The listing builds one solid part. Answer for the finished solid, in the listing's coordinates (mm). A direction names the side the tool comes from. Coordinates: 2 decimals unless noted, no trailing zeros. Order: outer loops, then holes, each group sorted by start corner. A loop starts at its lowest first (then second) coordinate and runs counter-clockwise, first axis right, second up.
```python
from build123d import *

# Parameters (mm, degrees)
SKETCH1_W           = 112.5
SKETCH1_H           = 21.6
SKETCH1_R           = 2
BOSS_EXTRUDE1_DEPTH = 13
SKETCH2_W           = 8
SKETCH2_H           = 21.6
CUT_EXTRUDE1_DEPTH  = 5.8
FILLET1_R           = 1


with BuildPart() as part:
    # Sketch1 → Boss-Extrude1 (new body)
    with BuildSketch(Plane.XY):
        Rectangle(SKETCH1_W, SKETCH1_H)
        with Locations(Location((-52.5, 4, 0), (0, 0, 180))):
            Circle(SKETCH1_R, mode=Mode.SUBTRACT)
        with Locations(Location((52.5, 4, 0), (0, 0, 180))):
            Circle(SKETCH1_R, mode=Mode.SUBTRACT)
        with Locations(Location((52.5, -4, 0), (0, 0, 180))):
            Circle(SKETCH1_R, mode=Mode.SUBTRACT)
        with Locations(Location((-52.5, -4, 0), (0, 0, 180))):
            Circle(SKETCH1_R, mode=Mode.SUBTRACT)
    extrude(amount=BOSS_EXTRUDE1_DEPTH)

    # Sketch2 → Cut-Extrude1 (cut)
    with BuildSketch(Plane.XY.offset(13)):
        with Locations((-42.75, 0)):
            Rectangle(SKETCH2_W, SKETCH2_H)
        with Locations((-52.25, 0)):
            Rectangle(SKETCH2_W, SKETCH2_H)
        with Locations((-33.25, 0)):
            Rectangle(SKETCH2_W, SKETCH2_H)
        with Locations((-23.75, 0)):
            Rectangle(SKETCH2_W, SKETCH2_H)
        with Locations((-14.25, 0)):
            Rectangle(SKETCH2_W, SKETCH2_H)
        with Locations((-4.75, 0)):
            Rectangle(SKETCH2_W, SKETCH2_H)
        with Locations((4.75, 0)):
            Rectangle(SKETCH2_W, SKETCH2_H)
        with Locations((14.25, 0)):
            Rectangle(SKETCH2_W, SKETCH2_H)
        with Locations((23.75, 0)):
            Rectangle(SKETCH2_W, SKETCH2_H)
        with Locations((33.25, 0)):
            Rectangle(SKETCH2_W, SKETCH2_H)
        with Locations((42.75, 0)):
            Rectangle(SKETCH2_W, SKETCH2_H)
        with Locations((52.25, 0)):
            Rectangle(SKETCH2_W, SKETCH2_H)
    extrude(amount=-CUT_EXTRUDE1_DEPTH, mode=Mode.SUBTRACT)

    # Fillet1
    fillet1_edges = [part.edges().sort_by_distance(p)[0] for p in [
        (47.5, 10.8, 13),
        (38, 10.8, 13),
        (28.5, 10.8, 13),
        (19, 10.8, 13),
        (9.5, 10.8, 13),
        (0, 10.8, 13),
        (-9.5, 10.8, 13),
        (-19, 10.8, 13),
        (-28.5, 10.8, 13),
        (-38, 10.8, 13),
        (-47.5, 10.8, 13),
        (-47.5, -10.8, 13),
        (-38, -10.8, 13),
        (-28.5, -10.8, 13),
        (-19, -10.8, 13),
        (-9.5, -10.8, 13),
        (0, -10.8, 13),
        (9.5, -10.8, 13),
        (19, -10.8, 13),
        (28.5, -10.8, 13),
        (38, -10.8, 13),
        (47.5, -10.8, 13),
    ]]
    fillet(fillet1_edges, radius=FILLET1_R)


solid = part.part
```
(1) Each of these flat-tipped pins is pushed along its axis until it touches: pin 1 Ø4 at (x, y) = (-44, 0.5) entering from +Z; pin 2 Ø1.7 at (y, z) = (-3.5, 8.5) entering from -X; pin 3 Ø2 at (x, y) = (10, -1) entering from -Z; pin 4 Ø1.7 at (y, z) = (-1, 9.5) entering from +X. Where does it stop, or does it pass through?
(2) The mould has two halves that part along X. Classify faces 4 (the face through (56.25, 0, 4)), 5 (the face through (43, 0, 7.2)), 6 (the face through (52, 0, 7.2)): released by +X, released by -X, zero draft, split by the parting line, or undercut.
(3) Find section C-C (z = 11). Give the number of separate pieces and of enclosed holes in the cut face, and give its area (3 significant figures).
(4) For faces 1 (the face through (-52, 0, 7.2)), 2 (the face through (-43, 0, 7.2)), 3 (the face through (-1, -10.8, 3)), determine the directions among +Z, -Z, +X, -X, +Y, -Y from which every point of the face is accessible in a straight line to the end or side of a thin tool.
(5) Consider line 1 (X direction, y = 4, z = 2.5); line 2 (Y direction, x = 52.5, z = 4.25); line 3 (X direction, y = 3.5, z = 6.5). Determine where each line is inside the solid, lowest interval first.
(6) Find section A-A (z = 2). Write down the section's boundary in (x, y).
(7) Find section B-B (x = 52.5). Write down the section's boundary in (y, z).
Findings below:
1. pin 1: stops at z = 7.2
1. pin 2: stops at x = -48.25
1. pin 3: stops at z = 0
1. pin 4: stops at x = 48.25
2. face 4: released by +X
2. face 5: undercut
2. face 6: zero draft
3. separate pieces: 11
3. enclosed holes: 0
3. area: 356 mm2
4. face 1: +Z, -X, +Y, -Y
4. face 2: +Z, +Y, -Y
4. face 3: +Z, -Z, +X, -X, -Y
5. line 1: x = -56.25 to -54.5, -50.5 to 50.5, 54.5 to 56.25
5. line 2: y = -10.8 to -6, -2 to 2, 6 to 10.8
5. line 3: x = -56.25 to -54.44, -50.56 to 50.56, 54.44 to 56.25
6. outline: (-56.25, -10.8) - (56.25, -10.8) - (56.25, 10.8) - (-56.25, 10.8) - close; hole circle Ø4 at (-52.5, -4); hole circle Ø4 at (-52.5, 4); hole circle Ø4 at (52.5, -4); hole circle Ø4 at (52.5, 4)
7. outline: (-10.8, 0) - (-6, 0) - (-6, 7.2) - (-10.8, 7.2) - close; (-2, 0) - (2, 0) - (2, 7.2) - (-2, 7.2) - close; (6, 0) - (10.8, 0) - (10.8, 7.2) - (6, 7.2) - close
